```python
from build123d import *

# Parameters (mm, degrees)
PAD015_DEPTH    = 3
PAD016_DEPTH    = 2
PAD017_DEPTH    = 15
POCKET009_DEPTH = 5
POCKET010_DEPTH = 2


with BuildPart() as part:
    # Sketch031 → Pad015 (new body)
    with BuildSketch(Plane(origin=(0, 0, 0), x_dir=(-1, 0, 0), z_dir=(0, 1, 0))):
        with BuildLine():
            Line((15, 3.2565168385), (15, 20.2565168385))
            Line((15, 20.2565168385), (0, 20.2565168385))
            Line((0, 20.2565168385), (0, 15.9565168385))
            ThreePointArc((0, 7.5565168385), (4.2, 11.7565168385), (0, 15.9565168385))
            Line((0, 7.5565168385), (0, 3.2565168385))
            Line((0, 3.2565168385), (15, 3.2565168385))
        make_face()
    pad015 = extrude(amount=PAD015_DEPTH)

    # Sketch032 (on Face3 of Pad015) → Pad016 (join)
    with BuildSketch(Plane(origin=(-15, 0, 0), x_dir=(0, 0, -1), z_dir=(-1, 0, 0))):
        Polygon((-3.2565168385, -3), (-3.2565168385, -22.8149545762), (-20.2565168385, -13), (-20.2565168385, -3), align=None)
    pad016 = extrude(amount=-PAD016_DEPTH)

    # Sketch034 (on Face11 of Pad016) → Pad017 (join)
    with BuildSketch(Plane(origin=(-15, 0, 0), x_dir=(0, 0, -1), z_dir=(-1, 0, 0))):
        Polygon((-20.2565168385, -13), (-20.2565168385, -17.6188021535), (-3.2565168385, -27.4337567297), (-3.2565168385, -22.8149545762), align=None)
    pad017 = extrude(amount=-PAD017_DEPTH)

    # Sketch035 (on Face16 of Pad017) → Pocket009 (cut)
    with BuildSketch(Plane(origin=(0, 21.9854307023, 12.6932943342), x_dir=(1, 0, 0), z_dir=(0, 0.8660254038, 0.5))):
        with BuildLine():
            ThreePointArc((0, 2.9722964019), (-4.2, -1.2277035981), (0, -5.4277035981))
            Line((0, -5.4277035981), (0, 2.9722964019))
        make_face()
    pocket009 = extrude(amount=-POCKET009_DEPTH, mode=Mode.SUBTRACT)

    # Sketch036 (on Face14 of Pocket009) → Pocket010 (cut)
    with BuildSketch(Plane(origin=(0, 18.5213290872, 10.6932943342), x_dir=(1, 0, 0), z_dir=(0, -0.8660254038, -0.5))):
        Polygon((3.7527767497, 7.7277035981), (-3.7527767497, 7.7277035981), (-7.5055534995, 1.2277035981), (-3.7527767497, -5.2722964019), (3.7527767497, -5.2722964019), (7.5055534995, 1.2277035981), align=None)
    pocket010 = extrude(amount=-POCKET010_DEPTH, mode=Mode.SUBTRACT)

    # Mirrored008: Pad015, Pad016, Pad017, Pocket009, Pocket010 across Sketch031 V_Axis
    add(pad015.mirror(Plane(origin=(0, 0, 0), x_dir=(0, 1, 0), z_dir=(-1, 0, 0))))
    add(pad016.mirror(Plane(origin=(0, 0, 0), x_dir=(0, 1, 0), z_dir=(-1, 0, 0))))
    add(pad017.mirror(Plane(origin=(0, 0, 0), x_dir=(0, 1, 0), z_dir=(-1, 0, 0))))
    add(pocket009.mirror(Plane(origin=(0, 0, 0), x_dir=(0, 1, 0), z_dir=(-1, 0, 0))), mode=Mode.SUBTRACT)
    add(pocket010.mirror(Plane(origin=(0, 0, 0), x_dir=(0, 1, 0), z_dir=(-1, 0, 0))), mode=Mode.SUBTRACT)


solid = part.part
```
Can you work these out from the model? Positions are in its coordinate system, mm. A direction names the side the tool comes from. Round coordinates to 2 decimals unless told otherwise and drop trailing zeros. Loops run counter-clockwise (first coordinate to the right, second up) from the corner with the lowest first, then second, coordinate; pieces in that order, holes last. Notation, with made-up numbers: M 66,83.25 L 80,83.25 A15 cw 80,96.25 Z; hole C 53.5,-19.5 d11. An arc over 180 degrees is marked long. Write item = value, one per line. Start each with the question number.
(1) Suppose I cut it at B-B on y = 11.75. Write out the boundary of the cut face in (x, z).
(2) Suppose I cut it at A-A on x = -12.25. Write out the boundary of the cut face in (y, z), plus the area to 3 significant figures.
(3) I'm going to push flat-ended pins straight in: P1, Ø1.5, axis at x = -9, z = 10, coming from the +Y side; P2, Ø5, axis at x = 0, z = 9, coming from the +Y side; P3, Ø2, axis at x = -4, z = 12.5, coming from the +Y side. Where does each tip first touch, or does it pass through?
(4) I need wall thicknesses on line 1 along X through (y, z) = (12.75, 4.75); line 2 along Y through (x, z) = (-11, 4.5); line 3 along Y through (x, z) = (6, 10.75). Which ranges of each line are inside material? Lowest first, please.
(5) If we mould it in two halves opening along X, with no side actions, what happens to faces 6 (the face through (15, 10, 12)), 7 (the face through (-3.23, 18.15, 15.34)), 8 (the face through (-15, 10, 12))? For each: released by +X, released by -X, zero draft, split by the parting line, or undercut.
(6) Which directions (+Z, -Z, +X, -X, +Y, -Y) give clear straight access to the entire face, cutting with the end or side of a thin tool? Please do faces 1 (the face through (0.05, 15.51, 17.88)), 2 (the face through (-3, 3, 16)), 3 (the face through (0.05, 22.01, 6.62)), 4 (the face through (0, 23, 3.257)), 5 (the face through (0.21, 23.548, 9.987)).
(7) Suppose I cut it at D-D on x = -6.75. Write out the boundary of the cut face in (y, z).
(8) Suppose I cut it at C-C on x = -0.5. Write out the boundary of the cut face in (y, z), plus the area to 3 significant figures.
Answer block:
q1.outline = M -15,3.26 L -13,3.26 L -13,20.26 L -15,20.26 Z; M 13,3.26 L 15,3.26 L 15,20.26 L 13,20.26 Z
q2.outline = M 0,3.26 L 3,3.26 L 3,20.26 L 0,20.26 Z; M 13,20.26 L 22.81,3.26 L 27.43,3.26 L 17.62,20.26 Z
q2.area = 130 mm²
q3.P1 = 23.97
q3.P2 = 25.56
q3.P3 = 22.67
q4.line_1 = -15 to -13, 13 to 15
q4.line_2 = 0 to 3, 22.1 to 26.72
q4.line_3 = 0 to 3, 20.8 to 23.11
q5.face_6 = released by +X
q5.face_7 = undercut
q5.face_8 = released by -X
q6.face_1 = -Z
q6.face_2 = +Z, -Z
q6.face_3 = none
q6.face_4 = -Z, +X, -X, +Y, -Y
q6.face_5 = +Z, +X, -X, +Y
q7.outline = M 0,3.26 L 3,3.26 L 3,20.26 L 0,20.26 Z; M 13,20.26 L 17.25,12.89 L 18.99,13.89 L 20.29,11.62 L 18.56,10.62 L 22.81,3.26 L 27.43,3.26 L 17.62,20.26 Z
q8.outline = M 0,3.26 L 3,3.26 L 3,7.59 L 0,7.59 Z; M 0,15.93 L 3,15.93 L 3,20.26 L 0,20.26 Z; M 13,20.26 L 14.66,17.39 L 16.39,18.39 L 17.55,16.37 L 19.29,17.37 L 17.62,20.26 Z; M 21.16,6.13 L 22.81,3.26 L 27.43,3.26 L 23.46,10.15 L 21.72,9.15 L 22.89,7.13 Z
q8.area = 61.8 mm²
